Could you check a few things on this model? Use its own coordinates, in mm. A direction names the side the tool comes from. Give positions to 0.01 mm unless a question says otherwise; leave off trailing zeros. Write each loop counter-clockwise with the first axis right and the second up, starting at its lowest first coordinate (ties: lowest second). Pieces come first, ordered by that corner, then holes. Notation, with made-up numbers: M -30,26.25 L -17,26.25 A27 ccw -17,64.25 Z; hole C 36,24.25 d1. An arc over 180 degrees is marked long. Use one line per item in the form item = value.
from build123d import *

# Parameters (mm, degrees)
F0_W     = 508
F0_H     = 63.5
F0_W_2   = 506.476
F0_H_2   = 61.976
F1_DEPTH = 711.2
F2_DEPTH = 0.762
F3_R     = 50.8
F3_R_2   = 50.038
F4_DEPTH = 50.8
F5_DEPTH = 25.4


with BuildPart() as f1:
    # F0 (on Top) → F1 (new body)
    with BuildSketch(Plane.XY):
        Rectangle(F0_W, F0_H)
        Rectangle(F0_W_2, F0_H_2, mode=Mode.SUBTRACT)
    extrude(amount=F1_DEPTH)

    # F0 (on Top) → F2 (join)
    with BuildSketch(Plane.XY):
        Rectangle(F0_W_2, F0_H_2)
    extrude(amount=F2_DEPTH)

    # F3 (on face) → F4 (join)
    with BuildSketch(Plane(origin=(0, 31.75, 0), x_dir=(-1, 0, 0), z_dir=(0, 1, 0))):
        with Locations((0, 76.2)):
            Circle(F3_R)
        with Locations((0, 76.2)):
            Circle(F3_R_2, mode=Mode.SUBTRACT)
    extrude(amount=F4_DEPTH)

    # F3 (on face) → F5 (cut)
    with BuildSketch(Plane(origin=(0, 31.75, 0), x_dir=(-1, 0, 0), z_dir=(0, 1, 0))):
        with Locations((0, 76.2)):
            Circle(F3_R_2)
    extrude(amount=-F5_DEPTH, mode=Mode.SUBTRACT)


solid = f1.part
1) If I drill on L1, parallel to Y at x = 1, z = 203.5; L2, parallel to X at y = 16, z = 584.5; L3, parallel to Z at x = 0, y = 55, over which ranges is the centre line in solid material (lowest first)?
Checked values:
L1 = -31.75 to -30.99, 30.99 to 31.75
L2 = -254 to -253.24, 253.24 to 254
L3 = 25.4 to 26.16, 126.24 to 127
2) Thinking about a two-plate mould opening in X: for faces 1 (the flat face through (-4, 0, 0)), 2 (the cylindrical face through (11.012, 56.794, 26.608)), 3 (the flat face through (-253.238, 0, 351)), 4 (the flat face through (-4, 0, 0.762)), which applies, released by +X, released by -X, zero draft, split by the parting line, or undercut?
Checked values:
face_1 = zero draft
face_2 = split by the parting line
face_3 = undercut
face_4 = undercut
3) I want a section at A-A, the plane x = 0. Please give me the cut outline in (y, z), plus the area to 3 significant figures.
Checked values:
outline = M -31.75,0 L 31.75,0 L 31.75,25.4 L 82.55,25.4 L 82.55,26.16 L 30.99,26.16 L 30.99,0.76 L -30.99,0.76 L -30.99,711.2 L -31.75,711.2 Z; M 30.99,126.24 L 82.55,126.24 L 82.55,127 L 31.75,127 L 31.75,711.2 L 30.99,711.2 Z
area = 1,130 mm2
4) For faces 5 (the flat face through (254, 0, 351)), 6 (the flat face through (-4, 30.988, 351)), which set-ups out of +Z, -Z, +X, -X, +Y, -Y let a thin tool reach every point of the face, with its end or its side?
Checked values:
face_5 = +Z, -Z, +X, +Y, -Y
face_6 = +Z
5) I want a section at C-C, the plane y = -9. Please give me the cut outline in (x, z).
Checked values:
outline = M -254,0 L 254,0 L 254,711.2 L 253.24,711.2 L 253.24,0.76 L -253.24,0.76 L -253.24,711.2 L -254,711.2 Z
6) I want a section at D-D, the plane x = -171. Please give me the cut outline in (y, z), plus the area to 3 significant figures.
Checked values:
outline = M -31.75,0 L 31.75,0 L 31.75,711.2 L 30.99,711.2 L 30.99,0.76 L -30.99,0.76 L -30.99,711.2 L -31.75,711.2 Z
area = 1,130 mm2
7) I want a section at B-B, the plane z = 259. Please give me the cut outline in (x, y), plus the area to 3 significant figures.
Checked values:
outline = M -254,-31.75 L 254,-31.75 L 254,31.75 L -254,31.75 Z; hole M -253.24,-30.99 L 253.24,-30.99 L 253.24,30.99 L -253.24,30.99 Z
area = 869 mm2
8) For pin 1 Ø10 at (x, y) = (-8, 13) entering from -Z; pin 2 Ø2 at (x, y) = (10.5, 40) entering from -Z; pin 3 Ø4 at (x, y) = (146, -14) entering from +Z; pin 4 Ø2 at (x, y) = (149.5, 34) entering from -Z, each with a flat end and sliding along its axis, tell me the tip position at first contact or that it passes through.
Checked values:
pin_1 = 0
pin_2 = 26.3
pin_3 = 0.76
pin_4 = through
